Can you work these out from the model? Positions are in its coordinate system, mm. A direction names the side the tool comes from. Round coordinates to 2 decimals unless told otherwise and drop trailing zeros. Write each loop counter-clockwise with the first axis right and the second up, starting at its lowest first coordinate (ties: lowest second). Pieces come first, ordered by that corner, then holes.
Q1. If we section it at A-A (z = -2): Please give me the cut outline in (x, y).
Q2. Please list where these lines run through material, in increasing order: line 1 along Z through (x, y) = (-9.5, 13); line 2 along X through (y, z) = (41, 26.5); line 3 along Y through (x, z) = (-18, -56).
Q3. We'd pull the mould along Z, two halves only. Please class faces 6 (the cylindrical face through (-3.62, 81.19, 25.1)), 7 (the flat face through (-1, 2, -66)), 8 (the cylindrical face through (-24.14, 66.15, -28.46)): +Z half, -Z half, draft (parallel to the pull), parting line (faces both ways), or undercut.
Q4. For faces 1 (the flat face through (-35, 82.05, 28)), 2 (the flat face through (25, 45, 28)), 3 (the flat face through (-1, 5, -50)), 4 (the cylindrical face through (-3.62, 81.19, -25.1)), 5 (the cylindrical face through (-31.301, 2.465, 50.898)), which set-ups out of +Z, -Z, +X, -X, +Y, -Y let a thin tool reach every point of the face, with its end or its side?
Q5. If we section it at B-B (y = 9.5): Please give me the cut outline in (x, z).
Q6. If we section it at D-D (y = 55): Please give me the cut outline in (x, z), plus the area to 3 significant figures.
Q7. I'm going to push flat-ended pins straight in: pin 1 Ø5 at (x, y) = (26, 35.5) entering from +Z; pin 2 Ø2.5 at (y, z) = (83.5, -4.5) entering from -X; pin 3 Ø4 at (x, y) = (-0.5, 84.5) entering from -Z. Where does each tip first touch, or does it pass through?
Q8. If we section it at C-C (x = -9.5): Please give me the cut outline in (y, z), plus the area to 3 significant figures.
from build123d import *

# Parameters (mm, degrees)
SKETCH1_W               = 80
SKETCH1_H               = 40
SKETCH1_R               = 2.25
BOSS_EXTRUDE1_DEPTH     = 5
BOSS_EXTRUDE1_2_DEPTH   = 5
SKETCH2_W               = 80
SKETCH2_H               = 5
BOSS_EXTRUDE2_DEPTH     = 77.05
SKETCH3_W               = 43.85
SKETCH3_H               = 62
BOSS_EXTRUDE3_DEPTH     = 5
SKETCH5_W               = 29.85
SKETCH5_H               = 38
CUT_EXTRUDE2_DEPTH      = 10
CUT_EXTRUDE1_REACH      = 118.334
SKETCH4_R               = 1.3
FILLET1_R               = 3
FILLET2_R               = 3
CUT_EXTRUDE3_DEPTH      = 137.333057253
CUT_EXTRUDE3_DEPTH_BACK = 137.333057253
SKETCH6_W               = 50
SKETCH6_H               = 44.05
FILLET3_R               = 3


with BuildPart() as part:
    # Sketch1 → Boss-Extrude1 (new body)
    with BuildSketch(Plane(origin=(0, 0, 0), x_dir=(1, 0, 0), z_dir=(0, 1, 0))):
        with Locations((0, 46)):
            Rectangle(SKETCH1_W, SKETCH1_H)
        with Locations(Location((-30.625, 53.044055982, 0), (0, 0, 270))):
            Circle(SKETCH1_R, mode=Mode.SUBTRACT)
        with Locations(Location((30.625, 53.044055982, 0), (0, 0, 90))):
            Circle(SKETCH1_R, mode=Mode.SUBTRACT)
    extrude(amount=BOSS_EXTRUDE1_DEPTH)



with BuildPart() as body_2:
    # Sketch1 → Boss-Extrude1 2 (new body)
    with BuildSketch(Plane(origin=(0, 0, 0), x_dir=(1, 0, 0), z_dir=(0, 1, 0))):
        with Locations((0, -46)):
            Rectangle(SKETCH1_W, SKETCH1_H)
        with Locations(Location((30.625, -53.044055982, 0), (0, 0, 270))):
            Circle(SKETCH1_R, mode=Mode.SUBTRACT)
        with Locations(Location((-30.625, -53.044055982, 0), (0, 0, 90))):
            Circle(SKETCH1_R, mode=Mode.SUBTRACT)
    extrude(amount=BOSS_EXTRUDE1_2_DEPTH)


with BuildPart() as part_1:
    add(part.part)

    add(body_2.part)  # Boss-Extrude2 merges body 2
    # Sketch2 → Boss-Extrude2 (add)
    with BuildSketch(Plane(origin=(0, 5, 0), x_dir=(1, 0, 0), z_dir=(0, 1, 0))):
        with Locations((0, 28.5)):
            Rectangle(SKETCH2_W, SKETCH2_H)
        with Locations((0, -28.5)):
            Rectangle(SKETCH2_W, SKETCH2_H)
    extrude(amount=BOSS_EXTRUDE2_DEPTH)

    # Sketch3 → Boss-Extrude3 (add)
    with BuildSketch(Plane(origin=(0, 82.05, 0), x_dir=(1, 0, 0), z_dir=(0, 1, 0))):
        with Locations((-3.925, 0)):
            Rectangle(SKETCH3_W, SKETCH3_H)
    extrude(amount=BOSS_EXTRUDE3_DEPTH)

    # Sketch5 → Cut-Extrude2 (cut)
    with BuildSketch(Plane.XZ.offset(-82.05)):
        with Locations((-3.925, 0)):
            Rectangle(SKETCH5_W, SKETCH5_H)
    extrude(amount=-CUT_EXTRUDE2_DEPTH, mode=Mode.SUBTRACT)

    # Sketch4 → Cut-Extrude1 (cut, up to next)
    with BuildSketch(Plane(origin=(0, 87.05, 0), x_dir=(1, 0, 0), z_dir=(0, 1, 0)), mode=Mode.PRIVATE) as cut_extrude1_sk1:
        with Locations(Location((-23, 20, 0), (0, 0, 270))):
            Circle(SKETCH4_R)
    cut_extrude1_tool1 = extrude(cut_extrude1_sk1.sketch, amount=-CUT_EXTRUDE1_REACH, mode=Mode.PRIVATE) & part_1.part
    # Sketch4 → Cut-Extrude1 (cut, up to next)
    with BuildSketch(Plane(origin=(0, 87.05, 0), x_dir=(1, 0, 0), z_dir=(0, 1, 0)), mode=Mode.PRIVATE) as cut_extrude1_sk2:
        with Locations(Location((15, 20, 0), (0, 0, 270))):
            Circle(SKETCH4_R)
    cut_extrude1_tool2 = extrude(cut_extrude1_sk2.sketch, amount=-CUT_EXTRUDE1_REACH, mode=Mode.PRIVATE) & part_1.part
    # Sketch4 → Cut-Extrude1 (cut, up to next)
    with BuildSketch(Plane(origin=(0, 87.05, 0), x_dir=(1, 0, 0), z_dir=(0, 1, 0)), mode=Mode.PRIVATE) as cut_extrude1_sk3:
        with Locations(Location((15, -20, 0), (0, 0, 270))):
            Circle(SKETCH4_R)
    cut_extrude1_tool3 = extrude(cut_extrude1_sk3.sketch, amount=-CUT_EXTRUDE1_REACH, mode=Mode.PRIVATE) & part_1.part
    # Sketch4 → Cut-Extrude1 (cut, up to next)
    with BuildSketch(Plane(origin=(0, 87.05, 0), x_dir=(1, 0, 0), z_dir=(0, 1, 0)), mode=Mode.PRIVATE) as cut_extrude1_sk4:
        with Locations(Location((-23, -20, 0), (0, 0, 270))):
            Circle(SKETCH4_R)
    cut_extrude1_tool4 = extrude(cut_extrude1_sk4.sketch, amount=-CUT_EXTRUDE1_REACH, mode=Mode.PRIVATE) & part_1.part
    add(cut_extrude1_tool1.solids().sort_by_distance((-23, 87.05, -20))[0], mode=Mode.SUBTRACT)
    add(cut_extrude1_tool2.solids().sort_by_distance((15, 87.05, -20))[0], mode=Mode.SUBTRACT)
    add(cut_extrude1_tool3.solids().sort_by_distance((15, 87.05, 20))[0], mode=Mode.SUBTRACT)
    add(cut_extrude1_tool4.solids().sort_by_distance((-23, 87.05, 20))[0], mode=Mode.SUBTRACT)

    # Fillet1
    fillet1_edges = [part_1.edges().sort_by_distance(p)[0] for p in [
        (0, 5, -31),
        (-3.925, 82.05, -26),
        (-3.925, 82.05, 26),
        (0, 5, 31),
    ]]
    fillet(fillet1_edges, radius=FILLET1_R)

    # Fillet2
    fillet2_edges = [part_1.edges().sort_by_distance(p)[0] for p in [
        (18, 82.05, -28.5),
        (-25.85, 82.05, -28.5),
        (-25.85, 82.05, 28.5),
        (18, 82.05, 28.5),
    ]]
    fillet(fillet2_edges, radius=FILLET2_R)

    # Sketch6 → Cut-Extrude3 (cut, two sides: drawn at the far end of the back side and taken through both)
    with BuildSketch(Plane.XY.offset(31).offset(-CUT_EXTRUDE3_DEPTH_BACK)):
        with Locations((0, 45.025)):
            Rectangle(SKETCH6_W, SKETCH6_H)
    extrude(amount=CUT_EXTRUDE3_DEPTH + CUT_EXTRUDE3_DEPTH_BACK, mode=Mode.SUBTRACT)

    # Fillet3
    fillet3_edges = [part_1.edges().sort_by_distance(p)[0] for p in [
        (-25, 67.05, -28.5),
        (-25, 67.05, 28.5),
        (-25, 23, -28.5),
        (-25, 23, 28.5),
        (25, 23, -28.5),
        (25, 23, 28.5),
        (25, 67.05, -28.5),
        (25, 67.05, 28.5),
        (-18.85, 84.55, -19),
        (-18.85, 84.55, 19),
        (11, 84.55, 19),
        (11, 84.55, -19),
    ]]
    fillet(fillet3_edges, radius=FILLET3_R)


solid = part_1.part
A:
1. outline: (-25.85, 82.05) - (-18.85, 82.05) - (-18.85, 87.05) - (-25.85, 87.05) - close; (11, 82.05) - (18, 82.05) - (18, 87.05) - (11, 87.05) - close
2. line 1: z = -31 to -26, 26 to 31
2. line 2: x = -40 to -25, 25 to 40
2. line 3: y = 0 to 5
3. face 6: undercut
3. face 7: -Z half
3. face 8: draft
4. face 1: +Z, -Z, -X, +Y
4. face 2: +Z, -Z
4. face 3: -Z, +X, -X, +Y
4. face 4: +X, -X, -Y
4. face 5: +Y, -Y
5. outline: (-40, -31) - (40, -31) - (40, -26) - (-40, -26) - close; (-40, 26) - (40, 26) - (40, 31) - (-40, 31) - close
6. outline: (-40, -31) - (-25, -31) - (-25, -26) - (-40, -26) - close; (-40, 26) - (-25, 26) - (-25, 31) - (-40, 31) - close; (25, -31) - (40, -31) - (40, -26) - (25, -26) - close; (25, 26) - (40, 26) - (40, 31) - (25, 31) - close
6. area: 300 mm2
7. pin 1: stops at z = 31
7. pin 2: stops at x = -25.85
7. pin 3: stops at z = -31
8. outline: (0, -66) - (5, -66) - (5, -34) arc R3 cw to (8, -31) - (23, -31) - (23, -26) - (0, -26) - close; (0, 26) - (23, 26) - (23, 31) - (8, 31) arc R3 cw to (5, 34) - (5, 66) - (0, 66) - close; (67.05, -31) - (87.05, -31) - (87.05, -19) - (82.05, -19) - (82.05, -23) arc R3 cw to (79.05, -26) - (67.05, -26) - close; (67.05, 26) - (79.05, 26) arc R3 cw to (82.05, 23) - (82.05, 19) - (87.05, 19) - (87.05, 31) - (67.05, 31) - close
8. area: 858 mm2
